Part model, mm, in its own coordinate system. Face numbers are marked on the shaded views. A direction names the side the tool comes from. Round coordinates to 2 decimals unless told otherwise and drop trailing zeros. Loops run counter-clockwise (first coordinate to the right, second up) from the corner with the lowest first, then second, coordinate; pieces in that order, holes last. Notation, with made-up numbers: M -15.75,73 L -4.75,73 A12 ccw -4.75,86 Z; hole C 52.5,73 d7. An arc over 180 degrees is marked long. Answer as CSV lines item,"result". Start each with the question number.
Item 1: Drop flat-ended pins along their axis: pin 1 Ø6 at (x, y) = (9.5, -158.5) entering from -Z; pin 2 Ø2 at (x, y) = (14, -67) entering from +Z; pin 3 Ø11 at (x, y) = (15.5, -138.5) entering from +Z. Give the stop position or say it passes through.
Item 2: Mould opens along Y. For the marked faces 3, 4 and 5 say: pulls with the +Y half, pulls with the -Y half, needs draft (parallel to the pull), parting line crosses it, or undercut.
Item 3: Band-saw the part on B-B (y = -70). Give the cut face in (x, z), and give its area (3 significant figures).
Item 4: Which spindle directions (+Z, -Z, +X, -X, +Y, -Y) get a long thin tool onto all of the face, cutting with end or side? Do the marked faces 1 and 2. Say none if no direction does.
Item 5: Band-saw the part on C-C (z = 54). Give the cut face in (x, y), and give its area (3 significant figures).
Item 6: Wall check: line 1 (Y direction, x = 11, z = -49); line 2 (Y direction, x = 5, z = 2); line 3 (Z direction, x = 3, y = -140). Give the ranges that are in metal, low to high.
Item 7: Band-saw the part on D-D (x = 19.5). Count the separate pieces of the cut face and the enclosed holes in it, and give its area (3 significant figures).
Item 8: Band-saw the part on A-A (z = -20). Give the cut face in (x, y), and give its area (3 significant figures).
```python
from build123d import *

# Parameters (mm, degrees)
F0_R        = 71.6651662247
F1_DEPTH    = 21.844
F2_T        = 2.54
F2_T3_DEPTH = 26.924


# Not quite as in the source:
# - a shell that OpenCascade refuses in one call is made with other operations: the cavity is built on its own and cut out
# - a feature names something its author has since deleted; it is built from what else it names


with BuildPart() as f1:
    # F0 (on Right) → F1 (new body)
    with BuildSketch(Plane.YZ):
        with Locations((-115.809135139, -7.7714063227)):
            Circle(F0_R)
        with BuildLine():
            ThreePointArc((-108.3759665489, 16.3117386401), (-100.4681563218, 38.9034837812), (-94.1200479865, 15.824880451))
            Line((-94.1200479865, 15.824880451), (-81.7305743694, 0))
            Line((-81.7305743694, 0), (-64.600661397, 0))
            Line((-64.600661397, 0), (-64.600661397, -11.2849194556))
            Line((-64.600661397, -11.2849194556), (-89.6177664399, -11.2849194556))
            Line((-89.6177664399, -11.2849194556), (-101.0896414518, 0))
            Line((-101.0896414518, 0), (-108.967371285, -27.4995788932))
            Line((-108.967371285, -27.4995788932), (-86.5627974272, -71.233086288))
            Line((-86.5627974272, -71.233086288), (-97.011906829, -76.5861406686))
            Line((-97.011906829, -76.5861406686), (-119.9753677787, -31.7616911776))
            Line((-119.9753677787, -31.7616911776), (-125.7533729076, -46.8470752239))
            Line((-125.7533729076, -46.8470752239), (-152.9145538807, -46.8470752239))
            Line((-152.9145538807, -46.8470752239), (-156.1464071274, -46.8470752239))
            Line((-156.1464071274, -46.8470752239), (-169.7414368391, -46.8470752239))
            Line((-169.7414368391, -46.8470752239), (-169.7414368391, -36.2966917455))
            Line((-169.7414368391, -36.2966917455), (-156.1464071274, -36.2966917455))
            Line((-156.1464071274, -36.2966917455), (-134.1130137444, -36.2966917455))
            Line((-134.1130137444, -36.2966917455), (-129.4415742159, -11.2849194556))
            Line((-129.4415742159, -11.2849194556), (-118.9312636852, 4.8525910825))
            Line((-118.9312636852, 4.8525910825), (-128.7393420935, 4.8525910825))
            Line((-128.7393420935, 4.8525910825), (-139.9055675141, -12.2920099139))
            Line((-139.9055675141, -12.2920099139), (-149.2000942902, -6.2385134702))
            Line((-149.2000942902, -6.2385134702), (-131.8777501583, 15.824880451))
            Line((-131.8777501583, 15.824880451), (-108.3759665489, 16.3117386401))
        make_face(mode=Mode.SUBTRACT)
    extrude(amount=F1_DEPTH)

    # F2: shell of thickness 2.54, made by hand


with BuildPart() as f2_core1:
    # F2_t2: copy of F1
    add(f1.part)

    # the walls: a layer under each face that stays
    f2_faces = [f2_core1.faces().sort_by_distance(p)[0] for p in [
        (10.922, -187.4743013637, -7.7714063227),
        (10.922, -140.5389222243, 4.7931834904),
        (10.922, -144.5528309022, -9.2652616921),
        (10.922, -134.3224548038, -3.7197094157),
        (10.922, -123.8353028893, 4.8525910825),
        (10.922, -124.1864189506, -3.2161641866),
        (10.922, -131.7772939801, -23.7908056006),
        (10.922, -151.9272252917, -36.2966917455),
        (10.922, -169.7414368391, -41.5718834847),
        (10.922, -147.7474048734, -46.8470752239),
        (10.922, -122.8643703432, -39.3043832007),
        (10.922, -108.4936373039, -54.1739159231),
        (10.922, -91.7873521281, -73.9096134783),
        (10.922, -97.7650843561, -49.3663325906),
        (10.922, -105.0285063684, -13.7497894466),
        (10.922, -95.3537039459, -5.6424597278),
        (10.922, -77.1092139184, -11.2849194556),
        (10.922, -64.600661397, -5.6424597278),
        (10.922, -73.1656178832, 0),
        (10.922, -87.925311178, 7.9124402255),
        (10.922, -100.4681563218, 38.9034837812),
        (10.922, -120.1268583536, 16.0683095455),
        (0, -163.5859126221, -55.5481838059),
    ]]
    thicken(f2_faces, amount=-F2_T, mode=Mode.SUBTRACT)

    # F2_s4 → F2_t3 (cut)
    with BuildSketch(Plane.YZ.offset(-2.54)):
        Polygon((-149.1662539052, -6.2329149117), (-151.197922499, -4.6699847175), (-152.9114712381, -6.8525242483), (-150.5863045792, -8.3668980771), align=None)
        Polygon((-131.8572458078, 15.7838006118), (-133.8755783671, 17.3934092037), (-133.1328452619, 18.3394251098), (-131.9303569971, 18.3643356131), align=None)
        Polygon((-139.9129892573, -12.256863965), (-141.2917778031, -14.4203945208), (-139.1633931962, -15.8066048098), (-137.7771829073, -13.6782202029), align=None)
        Polygon((-129.3953221194, -11.3034448695), (-131.5699588227, -9.8987091667), (-131.8456535688, -10.3220103485), (-131.9383992614, -10.8185883585), align=None)
        Polygon((-169.7160368391, -36.3220917455), (-169.7414368391, -33.7566917455), (-172.2814368391, -33.7566917455), (-172.2814368391, -36.2966917455), align=None)
        Polygon((-169.7160368391, -46.8216752239), (-172.2814368391, -46.8470752239), (-172.2814368391, -49.3870752239), (-169.7414368391, -49.3870752239), align=None)
        Polygon((-125.7770925414, -46.8125901277), (-125.7533729076, -49.3870752239), (-124.0063031182, -49.3870752239), (-123.3814095297, -47.7555848463), align=None)
        Polygon((-97.0008817516, -76.5519534244), (-99.2725229084, -77.7442490147), (-98.1144145624, -80.0048650942), (-95.8537984829, -78.8467567481), align=None)
        Polygon((-86.5969846714, -71.2220612106), (-85.4046890811, -73.4937023674), (-83.1440730016, -72.3355940214), (-84.3021813477, -70.0749779419), align=None)
        Polygon((-89.5999540811, -11.2414120021), (-91.3990023244, -13.095664806), (-90.6576662231, -13.8249194556), (-89.6177664399, -13.8249194556), align=None)
        Polygon((-64.626061397, -11.2595194556), (-64.600661397, -13.8249194556), (-62.060661397, -13.8249194556), (-62.060661397, -11.2849194556), align=None)
        Polygon((-64.626061397, -0.0254), (-62.060661397, 0), (-62.060661397, 2.54), (-64.600661397, 2.54), align=None)
    extrude(amount=F2_T3_DEPTH, mode=Mode.SUBTRACT)


with BuildPart() as f1_1:
    add(f1.part)

    # what is left inside the walls is the cavity
    f2_cavity = [f2_core1.part.solids().sort_by_distance(p)[0] for p in [
        (15.409333, -139.586841, -72.651283),
        (21.8186, -150.371718, 17.74945),
    ]]
    add(f2_cavity, mode=Mode.SUBTRACT)


solid = f1_1.part
```
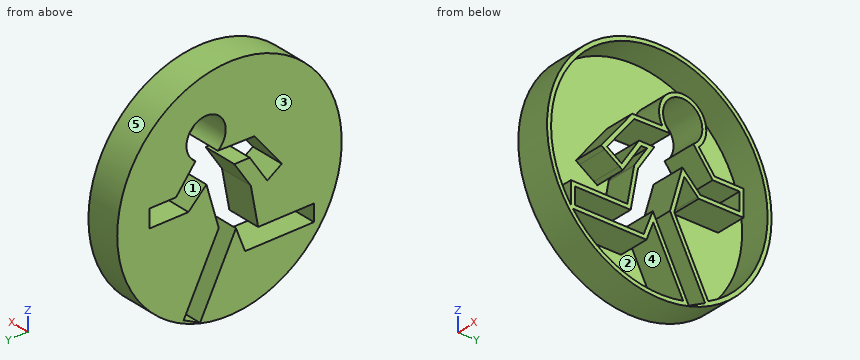
Answer block:
1,pin 1,"stops at z = -67.44"
1,pin 2,"stops at z = 45.62"
1,pin 3,"stops at z = 61.8"
2,face 3,"needs draft"
2,face 4,"undercut"
2,face 5,"parting line crosses it"
3,outline,"M 0,-62.88 L 21.84,-62.88 L 21.84,-59.54 L 2.54,-59.54 L 2.54,-13.82 L 21.84,-13.82 L 21.84,-11.28 L 0,-11.28 Z; M 0,0 L 21.84,0 L 21.84,2.54 L 2.54,2.54 L 2.54,44 L 21.84,44 L 21.84,47.34 L 0,47.34 Z"
3,area,"479 mm^2"
4,face 1,"+X, -X"
4,face 2,"+X"
5,outline,"M 0,-152.14 L 21.84,-152.14 L 21.84,-146.83 L 2.54,-146.83 L 2.54,-84.78 L 21.84,-84.78 L 21.84,-79.47 L 0,-79.47 Z"
5,area,"390 mm^2"
6,line 1,"y = -174.43 to -123.86, -114 to -111.14, -97.95 to -95.1, -60.32 to -57.19"
6,line 2,"y = -186.81 to -184.24, -145.96 to -142.73, -130.6 to -127.57, -123.82 to -120.79, -83.3 to -62.06, -47.38 to -44.81"
6,line 3,"z = -75.23 to -72.53, -49.39 to -46.85, -36.3 to -33.76, -15.26 to -12.23, 5.48 to 9.59, 56.98 to 59.69"
7,separate pieces,"1"
7,enclosed holes,"3"
7,area,"2,430 mm^2"
8,outline,"M 0,-186.42 L 21.84,-186.42 L 21.84,-183.84 L 2.54,-183.84 L 2.54,-133.65 L 21.84,-133.65 L 21.84,-131.07 L 0,-131.07 Z; M 0,-106.82 L 21.84,-106.82 L 21.84,-104.18 L 2.54,-104.18 L 2.54,-47.77 L 21.84,-47.77 L 21.84,-45.19 L 0,-45.19 Z"
8,area,"498 mm^2"
